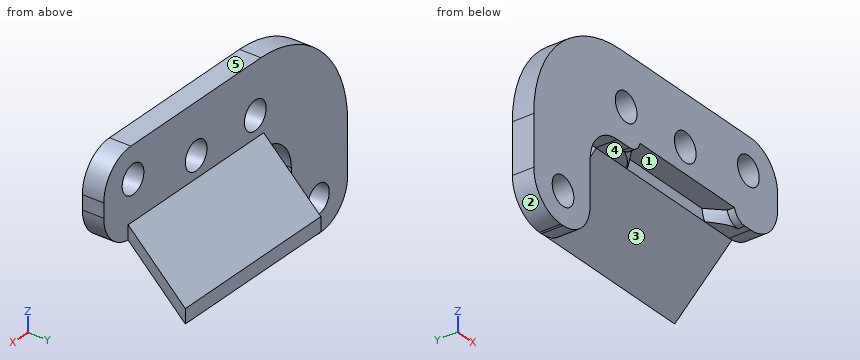
```python
from build123d import *

# Parameters (mm, degrees)
SKETCH1_W                = 45
SKETCH1_H                = 28
BOSS_EXTRUDE1_DEPTH      = 3
F_4_0_4_DIAMETER_HOLE1_D = 4
F_4_0_4_DIAMETER_HOLE2_D = 4
SKETCH10_W               = 34.6
SKETCH10_H               = 16
CUT_EXTRUDE2_DEPTH       = 3
FILLET2_R                = 5
FILLET3_R                = 16
BOSS_EXTRUDE2_START      = -5
BOSS_EXTRUDE2_DEPTH      = 25
SKETCH12_W               = 17.420537897
SKETCH12_H               = 1.5
CUT_EXTRUDE3_DEPTH       = 3
FILLET4_R                = 2
CHAMFER1_SIZE            = 2


with BuildPart() as part:
    # Sketch1 → Boss-Extrude1 (new body)
    with BuildSketch(Plane(origin=(0, 0, 0), x_dir=(1, 0, 0), z_dir=(0, 1, 0))):
        Rectangle(SKETCH1_W, SKETCH1_H)
    extrude(amount=BOSS_EXTRUDE1_DEPTH)

    # Ø4.0 (4) Diameter Hole1 (through all)
    with Locations(Plane(origin=(0, 3, 0), x_dir=(1, 0, 0), z_dir=(0, 1, 0))):
        with Locations((-17.1, 9.5), (17.1, -9.5)):
            Hole(F_4_0_4_DIAMETER_HOLE1_D / 2)

    # Ø4.0 (4) Diameter Hole2 (through all)
    with Locations(Plane(origin=(0, 3, 0), x_dir=(1, 0, 0), z_dir=(0, 1, 0))):
        with Locations((-5.45, -7), (5.45, -7)):
            Hole(F_4_0_4_DIAMETER_HOLE2_D / 2)

    # Sketch10 → Cut-Extrude2 (cut)
    with BuildSketch(Plane(origin=(0, 3, 0), x_dir=(1, 0, 0), z_dir=(0, 1, 0))):
        with Locations((5.2, 6)):
            Rectangle(SKETCH10_W, SKETCH10_H)
    extrude(amount=-CUT_EXTRUDE2_DEPTH, mode=Mode.SUBTRACT)

    # Fillet2
    fillet2_edges = [part.edges().sort_by_distance(p)[0] for p in [
        (-12.1, 1.5, -14),
        (22.5, 1.5, 2),
        (-12.1, 1.5, 2),
        (-22.5, 1.5, -14),
        (22.5, 1.5, 14),
    ]]
    fillet(fillet2_edges, radius=FILLET2_R)

    # Fillet3
    fillet3_edges = [part.edges().sort_by_distance(p)[0] for p in [
        (-22.5, 1.5, 14),
    ]]
    fillet(fillet3_edges, radius=FILLET3_R)

    # Sketch11 → Boss-Extrude2 (add)
    with BuildSketch(Plane(origin=(23, 0, 0), x_dir=(0, 0, -1), z_dir=(1, 0, 0)).offset(BOSS_EXTRUDE2_START)):
        Polygon((-4, 3), (4, 11), (6, 11), (-2, 3), align=None)
    extrude(amount=-BOSS_EXTRUDE2_DEPTH)

    # Sketch12 → Cut-Extrude3 (cut)
    with BuildSketch(Plane.XZ):
        with Locations((5.806845965, 2.75)):
            Rectangle(SKETCH12_W, SKETCH12_H)
    extrude(amount=-CUT_EXTRUDE3_DEPTH, mode=Mode.SUBTRACT)

    # Fillet4
    # the kernel refuses this fillet: 2 mm, written as the material it takes off along each edge
    with BuildSketch(Plane(origin=(-2.903422983, -4.841229183, 2), x_dir=(0, 0, 1), z_dir=(0, 1, 0))) as fillet4_piece_1:
        with BuildLine():
            CenterArc((2, -1.936491673), FILLET4_R, 104.477512186, 75.522487814)
            Line((0, -1.936491673), (0, 0))
            Line((0, 0), (1.5, 0))
        make_face()
    extrude(amount=7.841229183, mode=Mode.SUBTRACT)
    with BuildSketch(Plane(origin=(14.517114914, -4.841229183, 2), x_dir=(1, 0, 0), z_dir=(0, 1, 0))) as fillet4_piece_2:
        with BuildLine():
            CenterArc((1.936491673, -2), FILLET4_R, 90, 75.522487814)
            Line((0, -1.5), (0, 0))
            Line((0, 0), (1.936491673, 0))
        make_face()
    extrude(amount=7.841229183, mode=Mode.SUBTRACT)

    # Chamfer1
    # the kernel refuses this chamfer: 2 mm, written as the material it adds along each edge
    with BuildSketch(Plane(origin=(-4.839914656, 3, 4), x_dir=(-0.680858233566239, 0, 0.732415227712437), z_dir=(-0.732415227712437, 0, -0.680858233566239))) as chamfer1_piece_1_section:
        Polygon((2, -CHAMFER1_SIZE), (2 + CHAMFER1_SIZE, 0), (2, 0), align=None)
    chamfer1_piece_1 = revolve(axis=Axis((-4.839914656, 3, 4), (0, 1, 0)), revolution_arc=222.910744897, mode=Mode.PRIVATE)
    chamfer1_piece_1 = split(chamfer1_piece_1, bisect_by=Plane(origin=(-2.32351346, 2.593002324, 2), z_dir=(0, 0, 1)), keep=Keep.TOP, mode=Mode.PRIVATE)
    chamfer1_piece_1 = split(chamfer1_piece_1, bisect_by=Plane(origin=(-2.32351346, 2.593002324, 3.5), z_dir=(0, 0, -1)), keep=Keep.TOP, mode=Mode.PRIVATE)
    add(chamfer1_piece_1)
    with BuildSketch(Plane(origin=(16.453606588, 3, 4), x_dir=(0, 0, -1), z_dir=(1, 0, 0))) as chamfer1_piece_2_section:
        Polygon((2, -CHAMFER1_SIZE), (2 + CHAMFER1_SIZE, 0), (2, 0), align=None)
    chamfer1_piece_2 = revolve(axis=Axis((16.453606588, 3, 4), (0, 1, 0)), revolution_arc=222.910744897, mode=Mode.PRIVATE)
    chamfer1_piece_2 = split(chamfer1_piece_2, bisect_by=Plane(origin=(14.636969069, 2.019912547, 2), z_dir=(0, 0, 1)), keep=Keep.TOP, mode=Mode.PRIVATE)
    chamfer1_piece_2 = split(chamfer1_piece_2, bisect_by=Plane(origin=(14.636969069, 3.296842404, 3.703157596), z_dir=(0, -0.7071067811865511, -0.7071067811865439)), keep=Keep.TOP, mode=Mode.PRIVATE)
    add(chamfer1_piece_2)


solid = part.part
```
Model file for the job. Use its own axes, mm. Face numbers are marked on the shaded views. A direction names the side the tool comes from. Round coordinates to 2 decimals unless told otherwise and drop trailing zeros. Loops run counter-clockwise (first coordinate to the right, second up) from the corner with the lowest first, then second, coordinate; pieces in that order, holes last. Notation, with made-up numbers: M 14,-13 L 54,-13 A31 ccw 54,17 Z; hole C -32.5,74 d6. An arc over 180 degrees is marked long. Put each result on its own line as item: value. Start each with the question number.
Item 1: Mould opens along X. For the marked faces 1, 2 and 3 say: released by +X, released by -X, zero draft, split by the parting line, or undercut.
Item 2: Cut at D-D (z = 9.5). List the corners of the cut face in (x, y).
Item 3: Cut at B-B (z = -1). List the corners of the cut face in (x, y).
Item 4: Drill centre lines: line 1 along Z through (x, y) = (17.1, 0.6); line 2 along X through (y, z) = (2.45, -9.5); line 3 along Z through (x, y) = (4.5, 1.5). Where is each one in solid material? Low to high.
Item 5: 3-axis set-ups, long thin cutter, end or side, ignore diameter. For the marked faces 4 and 5: which of +Z, -Z, +X, -X, +Y, -Y reach the whole face in a straight line?
Item 6: Cut at C-C (y = 2.5). List the corners of the cut face in (x, z), then the cut area to 3 significant figures.
Item 7: Drop flat-ended pins along their axis: P1, Ø0.8, axis at x = 3, z = 2.5, coming from the -Y side; P2, Ø6, axis at x = 4.5, z = -8.5, coming from the -Y side; P3, Ø1.5, axis at x = 18, y = 3, coming from the -Z side. Give the stop position or say it passes through.
Item 8: Cut at A-A (x = 5.45). List the corners of the cut face in (y, z).
Answer block:
1. face 1: undercut
1. face 2: released by -X
1. face 3: zero draft
2. outline: M -17.62,0 L 15.1,0 L 15.1,3 L -17.62,3 Z; M 19.1,0 L 22.47,0 L 22.47,3 L 19.1,3 Z
3. outline: M -22.47,0 L -11.68,0 L -11.68,3 L -22.47,3 Z; M -7,6 L 18,6 L 18,8 L -7,8 Z
4. line 1: 2 to 7.5, 11.5 to 14
4. line 2: -22.47 to -19.1, -15.1 to -12.13
4. line 3: 3.5 to 5.24, 8.76 to 14
5. face 4: -Z, +X, -Y
5. face 5: +Z, +X, -X, +Y, -Y
6. outline: M -22.5,-9 A5 ccw -17.5,-14 L -17.1,-14 A5 ccw -12.1,-9 L -12.1,-3 A5 cw -7.1,2 L -1.97,2 A3.5 ccw -1.38,3.5 L 12.99,3.5 A3.5 ccw 13.58,2 L 17.5,2 A5 ccw 22.5,7 L 22.5,9 A5 ccw 17.5,14 L -6.5,14 A16 ccw -22.5,-2 Z; hole C -17.1,-9.5 d4; hole C -5.45,7 d4; hole C 5.45,7 d4; hole C 17.1,9.5 d4
6. area: 563 mm2
7. P1: y = 3
7. P2: y = 10.5
7. P3: z = 1.25
8. outline: M 0,3.5 L 3,3.5 L 3,2 L 11,-6 L 11,-4 L 3,4 L 3,5 L 0,5 Z; M 0,9 L 3,9 L 3,14 L 0,14 Z
